```python
from build123d import *

# Parameters (mm, degrees)
F0_R     = 6.751658
F1_DEPTH = 1
F2_DEPTH = 25
F3_R     = 1.5


with BuildPart() as f1:
    # F0 (on Front) → F1 (new body)
    with BuildSketch(Plane.XZ):
        with BuildLine():
            Line((-74.545912, -21.686205), (35.944755, -21.686205))
            ThreePointArc((35.944755, -21.686205), (43.12896, -18.71041), (46.104755, -11.526205))
            Line((46.104755, -11.526205), (46.104755, 40.112911))
            ThreePointArc((46.104755, 40.112911), (43.12896, 47.297116), (35.944755, 50.272911))
            Line((35.944755, 50.272911), (-74.545912, 50.272911))
            ThreePointArc((-74.545912, 50.272911), (-81.730116, 47.297116), (-84.705912, 40.112911))
            Line((-84.705912, 40.112911), (-84.705912, -11.526205))
            ThreePointArc((-84.705912, -11.526205), (-81.730116, -18.71041), (-74.545912, -21.686205))
        make_face()
        with Locations((-74.545912, -11.526205)):
            Circle(F0_R, mode=Mode.SUBTRACT)
        with Locations((35.944755, -11.526205)):
            Circle(F0_R, mode=Mode.SUBTRACT)
        with Locations((-74.545912, 40.112911)):
            Circle(F0_R, mode=Mode.SUBTRACT)
        with Locations((35.944755, 40.112912)):
            Circle(F0_R, mode=Mode.SUBTRACT)
    extrude(amount=-F1_DEPTH)

    # F0 (on Front) → F2 (join)
    with BuildSketch(Plane.XZ):
        with Locations((35.944755, 40.112912)):
            Circle(F0_R)
        with Locations((35.944755, -11.526205)):
            Circle(F0_R)
        with Locations((-74.545912, -11.526205)):
            Circle(F0_R)
        with Locations((-74.545912, 40.112911)):
            Circle(F0_R)
    extrude(amount=-F2_DEPTH)

    # F3
    f3_edges = [f1.edges().sort_by_distance(p)[0] for p in [
        (-81.29757, 25, 40.112911),
        (29.193097, 25, 40.112912),
        (29.193097, 25, -11.526205),
        (-81.29757, 25, -11.526205),
    ]]
    fillet(f3_edges, radius=F3_R)


solid = f1.part
```
Can you work these out from the model? Positions are in its coordinate system, mm. A direction names the side the tool comes from. Coordinates: 2 decimals unless noted, no trailing zeros. Order: outer loops, then holes, each group sorted by start corner. A loop starts at its lowest first (then second) coordinate and runs counter-clockwise, first axis right, second up. Notation, with made-up numbers: (51.5, -21.5) -> (58.5, -21.5) arc R24 ccw to (58.5, 5.5) -> close; hole circle Ø7 at (34.25, -8). An arc over 180 degrees is marked (long way). Write each question's results on one line, items separated by ' | '.
Item 1: If I drill on line 1 along X through (y, z) = (9, -11.5); line 2 along Z through (x, y) = (-74, 16); line 3 along Y through (x, z) = (2, 34), over which ranges is the centre line in solid material (lowest first)?
Results are:
line 1: -81.3 to -67.79, 29.19 to 42.7 | line 2: -18.26 to -4.8, 33.38 to 46.84 | line 3: 0 to 1
Item 2: Which directions (+Z, -Z, +X, -X, +Y, -Y) give clear straight access to the entire face, cutting with the end or side of a thin tool? Please do faces 1 (the face through (-20, 1, 15)), 2 (the face through (-81.651, 0.493, 47.376)).
Results are:
face 1: +Y | face 2: +Z, -X, +Y, -Y
Item 3: I want a section at B-B, the plane x = -31. Write out the boundary of the cut face in (y, z), then the cut area to 3 significant figures.
Results are:
outline: (0, -21.69) -> (1, -21.69) -> (1, 50.27) -> (0, 50.27) -> close | area: 72.0 mm²
Item 4: I want a section at A-A, the plane y = 5. Write out the boundary of the cut face in (x, z), then the cut area to 3 significant figures.
Results are:
outline: circle Ø13.5 at (-74.55, -11.53); circle Ø13.5 at (-74.55, 40.11); circle Ø13.5 at (35.94, -11.53); circle Ø13.5 at (35.94, 40.11) | area: 573 mm²
Item 5: I'm going to push flat-ended pins straight in: pin 1 Ø8 at (y, z) = (5.5, 8.5) entering from +X; pin 2 Ø12 at (x, z) = (-57, -1) entering from +Y; pin 3 Ø10 at (y, z) = (13, -11) entering from +X; pin 4 Ø1.5 at (x, z) = (8, -6) entering from -Y. Where does each tip first touch, or does it pass through?
Results are:
pin 1: through | pin 2: y = 1 | pin 3: x = 42.7 | pin 4: y = 0
Item 6: If we mould it in two halves opening along Z, with no side actions, what happens to faces 3 (the face through (-20, 0, 15)), 4 (the face through (43.05, 0.49, -18.79)), 5 (the face through (30.587, 12.092, -15.634))? For each: +Z half, -Z half, draft (parallel to the pull), parting line (faces both ways), or undercut.
Results are:
face 3: draft | face 4: -Z half | face 5: undercut
Item 7: I want a section at C-C, the plane z = 13.5. Write out the boundary of the cut face in (x, y).
Results are:
outline: (-84.71, 0) -> (46.1, 0) -> (46.1, 1) -> (-84.71, 1) -> close
